Design review of the part shown in the three views and the two pictorial views. Dimensions are in mm from the part's minimum x, y and z. A direction names the side the tool comes from. Round coordinates to 2 decimals unless told otherwise and drop trailing zeros. Write each loop counter-clockwise with the first axis right and the second up, starting at its lowest first coordinate (ties: lowest second). Pieces come first, ordered by that corner, then holes. Notation, with made-up numbers: (30, -18) -> (44, -18) arc R10 cw to (44, 0) -> close; hole circle Ø4 at (-34.75, 76). An arc over 180 degrees is marked (long way). Answer as a JSON object with one key per item and string values. Group by question number.
1) We need section B-B, the plane x = 3. Count the separate pieces of the cut face and the enclosed holes in it, then the cut area to 3 significant figures.
2) We need section D-D, the plane z = 22.5. Write out the cut boundary in (x, y).
3) Machinability: for the marked faces 1 and 2, which of the approach directions +Z, -Z, +X, -X, +Y, -Y give a long, thin tool a straight path to every point of the face, cutting with its end or side? Answer none if there is none.
4) Insertion check: pin 1 Ø1.5 at (x, z) = (4, 31) entering from -Y; pin 2 Ø3 at (y, z) = (3, 18.5) entering from +X. Each pin has a flat end and moves straight along its axis. Give the tip position at first contact, or say it passes through.
5) To check wall thickness, follow probe 1 along Z at (x, y) = (2.65, 3); probe 2 along Z at (x, y) = (2, 4); probe 3 along Z at (x, y) = (5, 3.25). State the ranges of each line that lie inside material, in increasing order. Write a range as [from, to].
6) We need section A-A, the plane z = 3.5. Write out the cut boundary in (x, y).
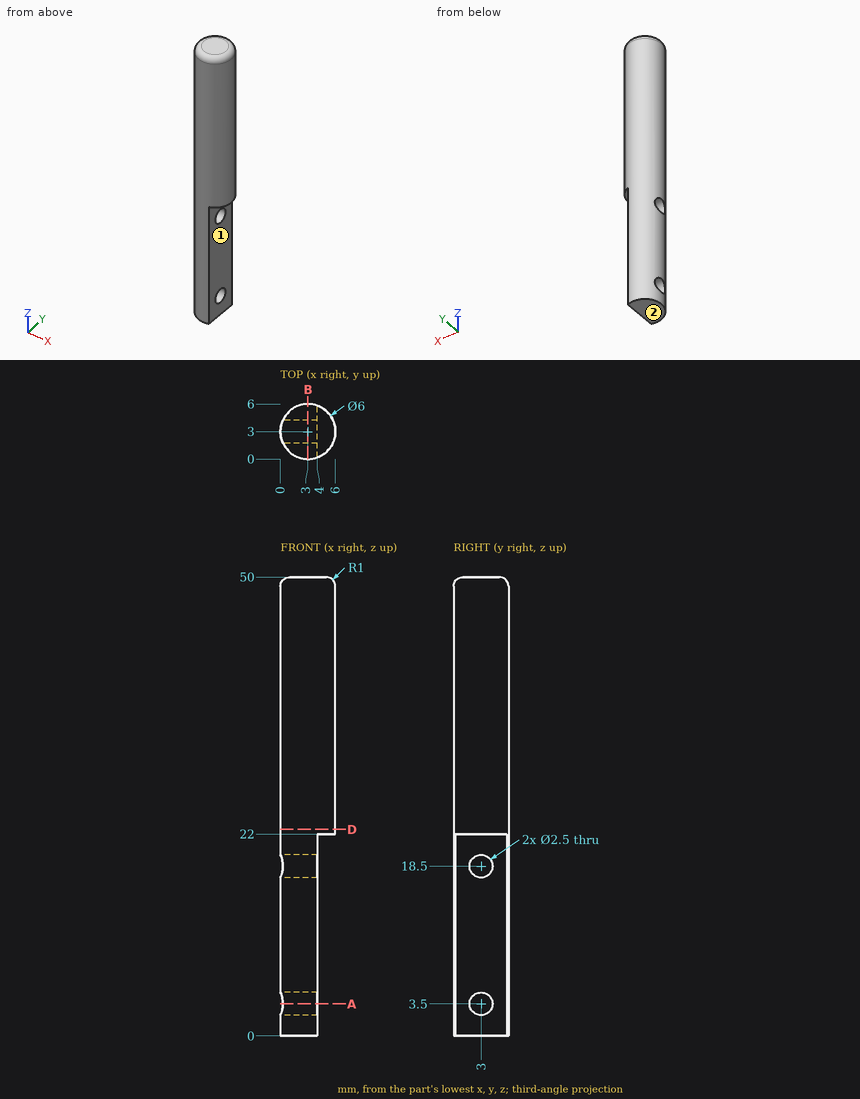
Here are the results:
{
 "1": {"separate pieces": "1", "enclosed holes": "2", "area": "290 mm^2"},
 "2": {"outline": "circle Ø6 at (3, 3)"},
 "3": {"face 1": "-Z, +X, +Y, -Y", "face 2": "-Z, +X, -X, +Y, -Y"},
 "4": {"pin 1": "stops at y = 0.01", "pin 2": "stops at x = 4"},
 "5": {"probe 1": "z = [0, 2.25], [4.75, 17.25], [19.75, 50]", "probe 2": "z = [0, 2.75], [4.25, 17.75], [19.25, 50]", "probe 3": "z = [22, 50]"},
 "6": {"outline": "(0.27, 1.75) arc R3 ccw to (4, 0.17) -> (4, 1.75) -> close; (0.27, 4.25) -> (4, 4.25) -> (4, 5.83) arc R3 ccw to start"}
}
